CAD build for the part. Positions are in the model's coordinates, mm. Coordinates: 2 decimals unless noted, no trailing zeros. Loops run counter-clockwise (first coordinate to the right, second up) from the corner with the lowest first, then second, coordinate; pieces in that order, holes last.
1) Saw through at B-B, the plane z = 12.5. Write the cut outline in (x, y).
2) Saw through at A-A, the plane y = -2.5. Write the cut outline in (x, z).
3) Saw through at C-C, the plane x = 30. Write the cut outline in (y, z).
4) Pin check, flat tips, straight feed: pin 1 Ø9 at (x, z) = (-65, 115) entering from -Y; pin 2 Ø4 at (x, y) = (2, -16) entering from +Z; pin 3 Ø1.5 at (y, z) = (1.5, -27.5) entering from +X; pin 4 Ø8.5 at (y, z) = (-15, 0) entering from +X. Stop position of each tip, or through.
5) Wall check: line 1 along X through (y, z) = (1, 115); line 2 along X through (y, z) = (1, -115); line 3 along Y through (x, z) = (25, -12.5). Give the ranges that are in metal, low to high.
```python
from build123d import *

# Parameters (mm, degrees)
SKETCH1_R           = 3.96875
BOSS_EXTRUDE1_DEPTH = 3
FILLET1_R           = 3
SKETCH9_R           = 4.7625
BOSS_EXTRUDE3_DEPTH = 5


with BuildPart() as part:
    # Sketch1 → Boss-Extrude1 (new body)
    with BuildSketch(Plane(origin=(0, 0, 0), x_dir=(1, 0, 0), z_dir=(0, 1, 0))):
        with BuildLine():
            Line((45, 105), (-45, 105))
            ThreePointArc((-45, 105), (-52.071067812, 107.928932188), (-55, 115))
            Line((-55, 115), (-55, 125))
            Line((-55, 125), (-75, 125))
            Line((-75, 125), (-75, 105))
            Line((-75, 105), (-65, 105))
            ThreePointArc((-65, 105), (-57.928932188, 102.071067812), (-55, 95))
            Line((-55, 95), (-55, -95))
            ThreePointArc((-55, -95), (-57.928932188, -102.071067812), (-65, -105))
            Line((-65, -105), (-75, -105))
            Line((-75, -105), (-75, -125))
            Line((-75, -125), (-54.202059137, -125))
            Line((-54.202059137, -125), (-54.202059137, -114.538060718))
            ThreePointArc((-54.202059137, -114.538060718), (-54.227177014, -113.870059928), (-54.202059137, -113.202059137))
            ThreePointArc((-54.202059137, -113.202059137), (-51.621839755, -107.580219382), (-46, -105))
            Line((-46, -105), (45, -105))
            ThreePointArc((45, -105), (52.04921496, -107.95078504), (55, -115))
            Line((55, -115), (55, -125))
            Line((55, -125), (75, -125))
            Line((75, -125), (75, -105))
            Line((75, -105), (65, -105))
            ThreePointArc((65, -105), (57.928932188, -102.071067812), (55, -95))
            Line((55, -95), (55, 95))
            ThreePointArc((55, 95), (57.928932188, 102.071067812), (65, 105))
            Line((65, 105), (75, 105))
            Line((75, 105), (75, 125))
            Line((75, 125), (55, 125))
            Line((55, 125), (55, 115))
            ThreePointArc((55, 115), (52.071067812, 107.928932188), (45, 105))
        make_face()
        with Locations(Location((-65, -115, 0), (0, 0, 270))):
            Circle(SKETCH1_R, mode=Mode.SUBTRACT)
        with Locations(Location((65, -115, 0), (0, 0, 270))):
            Circle(SKETCH1_R, mode=Mode.SUBTRACT)
        with Locations(Location((-65, 115, 0), (0, 0, 270))):
            Circle(SKETCH1_R, mode=Mode.SUBTRACT)
        with Locations(Location((65, 115, 0), (0, 0, 270))):
            Circle(SKETCH1_R, mode=Mode.SUBTRACT)
    extrude(amount=BOSS_EXTRUDE1_DEPTH)

    # Fillet1
    fillet1_edges = [part.edges().sort_by_distance(p)[0] for p in [
        (55, 1.5, -125),
        (75, 1.5, -125),
        (75, 1.5, -105),
        (75, 1.5, 105),
        (75, 1.5, 125),
        (55, 1.5, 125),
        (-54.202059137, 1.5, 125),
        (-75, 1.5, 125),
        (-75, 1.5, 105),
        (-75, 1.5, -105),
        (-75, 1.5, -125),
        (-55, 1.5, -125),
    ]]
    fillet(fillet1_edges, radius=FILLET1_R)

    # Sketch9 → Boss-Extrude3 (add, symmetric)
    with BuildSketch(Plane(origin=(0, 0, 0), x_dir=(0, 0, -1), z_dir=(1, 0, 0))):
        with BuildLine():
            Line((-15, 0), (15, 0))
            Line((15, 0), (15, -15.6))
            ThreePointArc((15, -15.6), (10.782337649, -25.782337649), (0.6, -30))
            Line((0.6, -30), (-0.6, -30))
            ThreePointArc((-0.6, -30), (-10.782337649, -25.782337649), (-15, -15.6))
            Line((-15, -15.6), (-15, 0))
        make_face()
        with Locations((0, -15)):
            Circle(SKETCH9_R, mode=Mode.SUBTRACT)
    extrude(amount=BOSS_EXTRUDE3_DEPTH, both=True)


solid = part.part
```
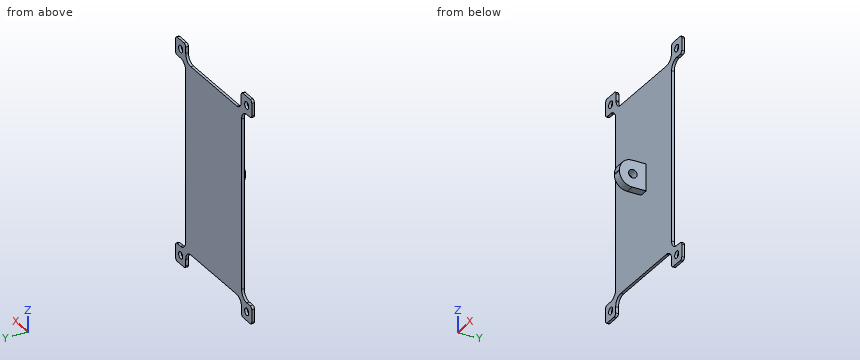
Data:
1. outline: (-55, 0) - (-5, 0) - (-5, -23.71) - (5, -23.71) - (5, 0) - (55, 0) - (55, 3) - (-55, 3) - close
2. outline: (-5, -15) - (5, -15) - (5, 15) - (-5, 15) - close
3. outline: (0, -105) - (3, -105) - (3, 105) - (0, 105) - close
4. pin 1: stops at y = 0
4. pin 2: stops at z = 15
4. pin 3: stops at x = 55
4. pin 4: passes through
5. line 1: x = -75 to -68.97, -61.03 to -54.2, 55 to 61.03, 68.97 to 75
5. line 2: x = -75 to -68.97, -61.03 to -55, 55 to 61.03, 68.97 to 75
5. line 3: y = 0 to 3
